Here's how the part is built. I have some questions about the finished solid (model axes, mm). Face numbers are marked on the shaded views. A direction names the side the tool comes from. Give positions to 0.01 mm unless a question says otherwise; leave off trailing zeros. Order: outer loops, then holes, each group sorted by start corner. A loop starts at its lowest first (then second) coordinate and runs counter-clockwise, first axis right, second up. Notation, with made-up numbers: (34.25, -30) -> (43.25, -30) arc R9 cw to (43.25, -24) -> close; hole circle Ø3 at (31, -37.75). An arc over 180 degrees is marked (long way). Write each question's results on one line, items separated by ' | '. Start each with the question number.
Q1. Imagine slicing it at C-C, the plane x = -10. Please give me the cut outline in (y, z), then the cut area to 3 significant figures.
Q2. Imagine slicing it at B-B, the plane z = 0. Please give me the cut outline in (x, y), then the cut area to 3 significant figures.
Q3. Imagine slicing it at A-A, the plane y = 0.5. Please give me the cut outline in (x, z), then the cut area to 3 significant figures.
Q4. I'm going to push flat-ended pins straight in: pin 1 (1.6 mm diameter, centred on x = 17.5, y = 1, fed in from +Z); pin 2 (1.2 mm diameter, centred on y = 2.5, z = 0, fed in from +X); pin 3 (3 mm diameter, centred on x = 16, z = 6.5, fed in from -Y). Where does each tip first touch, or does it pass through?
Q5. For the marked faces 1, 2 and 3, which set-ups out of +Z, -Z, +X, -X, +Y, -Y let a thin tool reach every point of the face, with its end or its side?
Q6. Imagine slicing it at D-D, the plane z = 5.5. Please give me the cut outline in (x, y), then the cut area to 3 significant figures.
Q7. I need wall thicknesses on line 1 along X through (y, z) = (0.95, 0); line 2 along Z through (x, y) = (-16, -2.5); line 3 along Y through (x, z) = (-7.5, -5.5). Which ranges of each line are inside material? Lowest first, please. Write a range as [from, to].
```python
from build123d import *

# Parameters (mm, degrees)
ESQUISSE1_R           = 1
ESQUISSE1_W           = 1
ESQUISSE1_H           = 10
BASE_DEPTH            = 1.5
ESQUISSE2_W           = 4
ESQUISSE2_H           = 5
SOIC_8_DEPTH          = 1.5
ESQUISSE3_W           = 8
ESQUISSE3_H           = 12
GROVE_CONNECTOR_DEPTH = 5.25


with BuildPart() as part:
    # Esquisse1 → Base (new body)
    with BuildSketch(Plane(origin=(0, 0, 0), x_dir=(1, 0, 0), z_dir=(0, 1, 0))):
        with BuildLine():
            Line((-20, -2), (-20, -10))
            Line((-20, -10), (-12.006445979, -10))
            ThreePointArc((-12.006445979, -10), (-10, -12.006445979), (-7.993554021, -10))
            Line((-7.993554021, -10), (8, -10))
            ThreePointArc((8, -10), (10, -8), (12, -10))
            Line((12, -10), (20, -10))
            Line((20, -10), (20, -2.006445979))
            ThreePointArc((20, -2.006445979), (22.006445979, 0), (20, 2.006445979))
            Line((20, 2.006445979), (20, 10))
            Line((20, 10), (12, 10))
            ThreePointArc((12, 10), (10, 8), (8, 10))
            Line((8, 10), (-8.006445979, 10))
            ThreePointArc((-8.006445979, 10), (-10, 11.993554021), (-11.993554021, 10))
            Line((-11.993554021, 10), (-20, 10))
            Line((-20, 10), (-20, 2))
            ThreePointArc((-20, 2), (-18, 0), (-20, -2))
        make_face()
        with Locations(Location((20, 0, 0), (0, 0, 270))):
            Circle(ESQUISSE1_R, mode=Mode.SUBTRACT)
        with Locations(Location((-10, 10, 0), (0, 0, 270))):
            Circle(ESQUISSE1_R, mode=Mode.SUBTRACT)
        with Locations(Location((-10, -10, 0), (0, 0, 270))):
            Circle(ESQUISSE1_R, mode=Mode.SUBTRACT)
        Rectangle(ESQUISSE1_W, ESQUISSE1_H, mode=Mode.SUBTRACT)
    extrude(amount=BASE_DEPTH)

    # Esquisse2 → SOIC-8 (add)
    with BuildSketch(Plane(origin=(0, 1.5, 0), x_dir=(1, 0, 0), z_dir=(0, 1, 0))):
        with Locations((10, 0)):
            Rectangle(ESQUISSE2_W, ESQUISSE2_H)
    extrude(amount=SOIC_8_DEPTH)

    # Esquisse3 → Grove connector (add)
    with BuildSketch(Plane(origin=(0, 0, 0), x_dir=(1, 0, 0), z_dir=(0, 1, 0))):
        with Locations((-15.044217332, 0)):
            Rectangle(ESQUISSE3_W, ESQUISSE3_H)
    extrude(amount=-GROVE_CONNECTOR_DEPTH)


solid = part.part
```
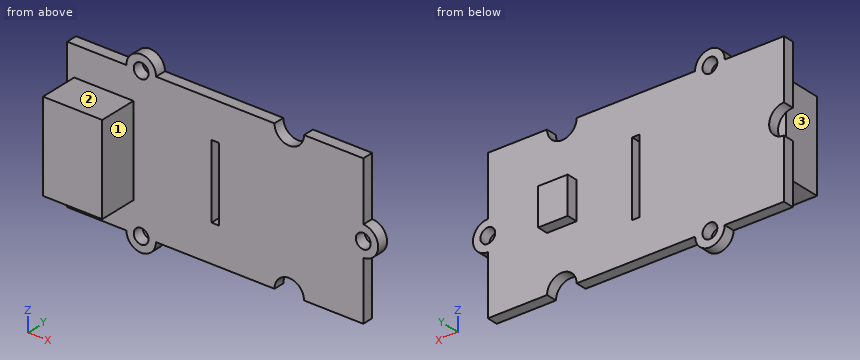
Geometry check:
1) outline: (0, -11.99) -> (1.5, -11.99) -> (1.5, -11) -> (0, -11) -> close; (0, -9) -> (1.5, -9) -> (1.5, 9) -> (0, 9) -> close; (0, 11) -> (1.5, 11) -> (1.5, 12.01) -> (0, 12.01) -> close | area: 30.0 mm²
2) outline: (-19.04, -5.25) -> (-11.04, -5.25) -> (-11.04, 0) -> (-0.5, 0) -> (-0.5, 1.5) -> (-18, 1.5) -> (-18, 0) -> (-19.04, 0) -> close; (0.5, 0) -> (19, 0) -> (19, 1.5) -> (12, 1.5) -> (12, 3) -> (8, 3) -> (8, 1.5) -> (0.5, 1.5) -> close; (21, 0) -> (22.01, 0) -> (22.01, 1.5) -> (21, 1.5) -> close | area: 104 mm²
3) outline: (-20, -10) -> (-11.99, -10) arc R1.99 ccw to (-8.01, -10) -> (8, -10) arc R2 cw to (12, -10) -> (20, -10) -> (20, -2.01) arc R2.01 ccw to (20, 2.01) -> (20, 10) -> (12, 10) arc R2 cw to (8, 10) -> (-7.99, 10) arc R2.01 ccw to (-12.01, 10) -> (-20, 10) -> (-20, 2) arc R2 cw to (-20, -2) -> close; hole circle Ø2 at (-10, -10); hole circle Ø2 at (-10, 10); hole (-0.5, -5) -> (0.5, -5) -> (0.5, 5) -> (-0.5, 5) -> close; hole circle Ø2 at (20, 0) | area: 781 mm²
4) pin 1: z = 10 | pin 2: x = 12 | pin 3: y = 0
5) face 1: +Z, -Z, +X, -Y | face 2: +Z, +X, -X, -Y | face 3: +Z, -Z, -X, -Y
6) outline: (-20, 0) -> (-19.04, 0) -> (-19.04, -5.25) -> (-11.04, -5.25) -> (-11.04, 0) -> (20, 0) -> (20, 1.5) -> (-20, 1.5) -> close | area: 102 mm²
7) line 1: [-18, -0.5], [0.5, 19], [21, 22.01] | line 2: [-6, 6] | line 3: [0, 1.5]
